The listing builds one solid part. Answer for the finished solid, in the listing's coordinates (mm). Face numbers are marked on the shaded views. A direction names the side the tool comes from. Round coordinates to 2 decimals unless told otherwise and drop trailing zeros. Write each loop counter-clockwise with the first axis right and the second up, starting at its lowest first coordinate (ties: lowest second). Pieces come first, ordered by that corner, then holes.
(1) Each of these flat-tipped pins is pushed along its axis until it touches: pin 1 Ø6 at (y, z) = (-15.5, 15.5) entering from +X; pin 2 Ø5 at (x, z) = (2.5, 15) entering from +Y; pin 3 Ø10 at (x, y) = (5, 2) entering from -Z; pin 4 Ø4 at (y, z) = (13, 13) entering from -X. Where does it stop, or does it pass through?
(2) Find the intervals of material crossed by probe 1 along Y at (x, z) = (0, 9); probe 2 along Z at (x, y) = (-12.5, 3.5); probe 3 along X at (y, z) = (5, 13), in increasing order.
(3) A cutting plane is placed at A-A, the plane z = 9.5. Give the vertices of the cut face in (x, y), and give its area (3 significant figures).
(4) The mould has two halves that part along X. Classify the marked faces 1, 2 and 3: +X half, -X half, draft (parallel to the pull), parting line (faces both ways), or undercut.
(5) For the marked faces 4 and 5, determine the directions among +Z, -Z, +X, -X, +Y, -Y from which every point of the face is accessible in a straight line to the end or side of a thin tool.
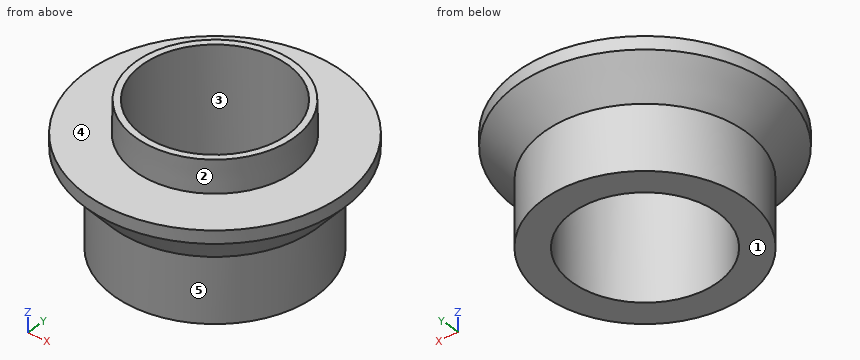
from build123d import *

# Parameters (mm, degrees)
SKETCH_10_R         = 15.75
EXTRUDE_5_DEPTH     = 10
SKETCH_12_R         = 20
SKETCH_14_R         = 20
EXTRUDE_6_DEPTH     = 2
SKETCH_16_R         = 12.35
SKETCH_15_R         = 12.45
SKETCH_17_R         = 11.35
CUT_EXTRUDE_3_DEPTH = 30


with BuildPart() as part:
    # 草图10 → 凸台-拉伸5 (new body)
    with BuildSketch(Plane.XY):
        Circle(SKETCH_10_R)
    extrude(amount=EXTRUDE_5_DEPTH)

    # 草图12 → section 0 of loft_5
    with BuildSketch(Plane.XY.offset(15), mode=Mode.PRIVATE) as loft_5_s0:
        Circle(SKETCH_12_R)
    # loft up to a face of the part (loft_5)
    loft([loft_5_s0.sketch, Face(Wire([part.edges().sort_by_distance((-10.781616918, 11.481255882, 10))[0]]))])

    # 草图14 → 凸台-拉伸6 (add)
    with BuildSketch(Plane.XY.offset(15)):
        Circle(SKETCH_14_R)
    extrude(amount=EXTRUDE_6_DEPTH)

    # 草图16 → 放样6 section 0
    with BuildSketch(Plane.XY.offset(22)):
        Circle(SKETCH_16_R)
    # 草图15 → 放样6 section 1
    with BuildSketch(Plane.XY.offset(17)):
        Circle(SKETCH_15_R)
    loft()

    # 草图17 → 切除-拉伸3 (cut)
    with BuildSketch(Plane.XY.offset(22)):
        Circle(SKETCH_17_R)
    extrude(amount=-CUT_EXTRUDE_3_DEPTH, mode=Mode.SUBTRACT)


solid = part.part
Solutions:
1. pin 1: stops at x = 15.61
1. pin 2: stops at y = 20
1. pin 3: passes through
1. pin 4: stops at x = -15.73
2. probe 1: y = -15.75 to -11.35, 11.35 to 15.75
2. probe 2: z = 0 to 17
2. probe 3: x = -17.6 to -10.19, 10.19 to 17.6
3. outline: circle Ø31.5 at (0, 0); hole circle Ø22.7 at (0, 0)
3. area: 375 mm2
4. face 1: draft
4. face 2: parting line
4. face 3: undercut
5. face 4: +Z
5. face 5: -Z
